```python
from build123d import *

# Parameters (mm, degrees)
SKETCH1_R             = 3.5
BOSS_EXTRUDE1_DEPTH   = 5
BOSS_EXTRUDE1_2_DEPTH = 5
BOSS_EXTRUDE1_3_DEPTH = 5
BOSS_EXTRUDE1_4_DEPTH = 5
SKETCH2_W             = 96.075
SKETCH2_H             = 46.545
BOSS_EXTRUDE3_DEPTH   = 1.5
SKETCH3_W             = 96.075
SKETCH3_H             = 46.545
SKETCH3_W_2           = 93.075
SKETCH3_H_2           = 43.545
BOSS_EXTRUDE4_DEPTH   = 10
FILLET1_R             = 3
FILLET2_R             = 1.5
FILLET3_R             = 2
FILLET4_R             = 0.5


with BuildPart() as part:
    # Sketch1 → Boss-Extrude1 (new body)
    with BuildSketch(Plane(origin=(0, 1.6, 0), x_dir=(1, 0, 0), z_dir=(0, 1, 0))):
        with Locations(Location((-41.5925, 16.8275, 0), (0, 0, 270))):
            Circle(SKETCH1_R)
    extrude(amount=BOSS_EXTRUDE1_DEPTH)



with BuildPart() as body_2:
    # Sketch1 → Boss-Extrude1 2 (new body)
    with BuildSketch(Plane(origin=(0, 1.6, 0), x_dir=(1, 0, 0), z_dir=(0, 1, 0))):
        with Locations(Location((-41.5925, -16.8275, 0), (0, 0, 270))):
            Circle(SKETCH1_R)
    extrude(amount=BOSS_EXTRUDE1_2_DEPTH)


with BuildPart() as body_3:
    # Sketch1 → Boss-Extrude1 3 (new body)
    with BuildSketch(Plane(origin=(0, 1.6, 0), x_dir=(1, 0, 0), z_dir=(0, 1, 0))):
        with Locations(Location((41.5925, -16.8275, 0), (0, 0, 270))):
            Circle(SKETCH1_R)
    extrude(amount=BOSS_EXTRUDE1_3_DEPTH)


with BuildPart() as body_4:
    # Sketch1 → Boss-Extrude1 4 (new body)
    with BuildSketch(Plane(origin=(0, 1.6, 0), x_dir=(1, 0, 0), z_dir=(0, 1, 0))):
        with Locations(Location((41.5925, 16.8275, 0), (0, 0, 270))):
            Circle(SKETCH1_R)
    extrude(amount=BOSS_EXTRUDE1_4_DEPTH)


with BuildPart() as part_1:
    add(part.part)

    add(body_2.part)  # Boss-Extrude3 merges body 2

    add(body_3.part)  # Boss-Extrude3 merges body 3

    add(body_4.part)  # Boss-Extrude3 merges body 4
    # Sketch2 → Boss-Extrude3 (add)
    with BuildSketch(Plane(origin=(0, 6.6, 0), x_dir=(1, 0, 0), z_dir=(0, 1, 0))):
        Rectangle(SKETCH2_W, SKETCH2_H)
    extrude(amount=-BOSS_EXTRUDE3_DEPTH)

    # Sketch3 → Boss-Extrude4 (add)
    with BuildSketch(Plane.XZ.offset(-5.1)):
        Rectangle(SKETCH3_W, SKETCH3_H)
        Rectangle(SKETCH3_W_2, SKETCH3_H_2, mode=Mode.SUBTRACT)
    extrude(amount=BOSS_EXTRUDE4_DEPTH)

    # Fillet1
    fillet1_edges = [part_1.edges().sort_by_distance(p)[0] for p in [
        (48.0375, 0.85, -23.2725),
        (48.0375, 0.85, 23.2725),
        (-48.0375, 0.85, 23.2725),
        (-48.0375, 0.85, -23.2725),
    ]]
    fillet(fillet1_edges, radius=FILLET1_R)

    # Fillet2
    fillet2_edges = [part_1.edges().sort_by_distance(p)[0] for p in [
        (46.5375, 0.1, -21.7725),
        (46.5375, 0.1, 21.7725),
        (-46.5375, 0.1, 21.7725),
        (-46.5375, 0.1, -21.7725),
    ]]
    fillet(fillet2_edges, radius=FILLET2_R)

    # Fillet3
    fillet3_edges = [part_1.edges().sort_by_distance(p)[0] for p in [
        (48.0375, 6.6, 0),
        (0, 6.6, -23.2725),
        (-48.0375, 6.6, 0),
        (0, 6.6, 23.2725),
        (47.158820344, 6.6, 22.393820344),
        (-47.158820344, 6.6, 22.393820344),
        (-47.158820344, 6.6, -22.393820344),
        (47.158820344, 6.6, -22.393820344),
    ]]
    fillet(fillet3_edges, radius=FILLET3_R)

    # Fillet4
    fillet4_edges = [part_1.edges().sort_by_distance(p)[0] for p in [
        (-46.5375, 5.1, 0),
        (0, 5.1, -21.7725),
        (46.5375, 5.1, 0),
        (0, 5.1, 21.7725),
        (46.098160172, 5.1, 21.333160172),
        (46.098160172, 5.1, -21.333160172),
        (-46.098160172, 5.1, 21.333160172),
        (-46.098160172, 5.1, -21.333160172),
    ]]
    fillet(fillet4_edges, radius=FILLET4_R)


solid = part_1.part
```
Source: CAD feature listing. Evaluate the final solid. Frame: model axes, mm. A direction names the side the tool comes from. Round coordinates to 2 decimals unless told otherwise and drop trailing zeros. Loops run counter-clockwise (first coordinate to the right, second up) from the corner with the lowest first, then second, coordinate; pieces in that order, holes last. Notation, with made-up numbers: M 23.5,46.5 L 73.5,46.5 A7 ccw 73.5,55.5 Z; hole C -2.75,49 d8. An arc over 180 degrees is marked long. Use a Markdown table: item, result. Add a question column.
1. Mould query, pull axis X, two halves, no side actions, for faces 3 (the cylindrical face through (47.467, 5.999, -0.284)), 4 (the cylindrical face through (-0.6, 6, -22.7)), 5 (the flat face through (46.538, 0, 0)), 6 (the flat face through (-48.038, 0, 0)). Classes: pulls with the +X half, pulls with the -X half, needs draft (parallel to the pull), parting line crosses it, or undercut.
2. Section query C-C on x = 12. Return the cut outline in (y, z).
3. Line query: line 1 (X direction, y = 0.25, z = 18); line 2 (Z direction, x = 32, y = 1.25); line 3 (X direction, y = 2.25, z = 14.5). Output: solid intervals per line, ascending.
4. Section query A-A on z = -2.5. Return the cut outline in (x, y).
5. Reachability of faces 1 (the cylindrical face through (-47.467, 5.999, 0.284)), 2 (the cylindrical face through (38.176, 3.326, 16.069)) from +Z, -Z, +X, -X, +Y, -Y: full face, straight path, thin tool, end or side. Return the list, or none.
6. Section query B-B on y = 2.5. Return the cut outline in (x, z).
7. Contact query for flat-ended pins moving along their axis: P1, Ø3.5, axis at x = -42, z = 16.5, coming from the -Y side; P2, Ø2, axis at x = -31, z = -2.5, coming from the -Y side; P3, Ø1.5, axis at y = 5.5, z = -15, coming from the +X side. Output: stop coordinate, or through.
8. Section query D-D on y = -3.25. Return the cut outline in (x, z).
Reported:
| question | item | result |
|---|---|---|
| 1 | face 3 | pulls with the +X half |
| 1 | face 4 | needs draft |
| 1 | face 5 | undercut |
| 1 | face 6 | pulls with the -X half |
| 2 | outline | M -4.9,-23.27 L 4.6,-23.27 A2 ccw 6.6,-21.27 L 6.6,21.27 A2 ccw 4.6,23.27 L -4.9,23.27 L -4.9,21.77 L 4.6,21.77 A0.5 cw 5.1,21.27 L 5.1,-21.27 A0.5 cw 4.6,-21.77 L -4.9,-21.77 Z |
| 3 | line 1 | x = -48.04 to -46.54, 46.54 to 48.04 |
| 3 | line 2 | z = -23.27 to -21.77, 21.77 to 23.27 |
| 3 | line 3 | x = -48.04 to -46.54, -44.21 to -38.98, 38.98 to 44.21, 46.54 to 48.04 |
| 4 | outline | M -48.04,-4.9 L -46.54,-4.9 L -46.54,4.6 A0.5 cw -46.04,5.1 L 46.04,5.1 A0.5 cw 46.54,4.6 L 46.54,-4.9 L 48.04,-4.9 L 48.04,4.6 A2 ccw 46.04,6.6 L -46.04,6.6 A2 ccw -48.04,4.6 Z |
| 5 | face 1 | +Z, -Z, -X, +Y |
| 5 | face 2 | -Y |
| 6 | outline | M -48.04,-20.27 A3 ccw -45.04,-23.27 L 45.04,-23.27 A3 ccw 48.04,-20.27 L 48.04,20.27 A3 ccw 45.04,23.27 L -45.04,23.27 A3 ccw -48.04,20.27 Z; C -41.59,-16.83 d7; C -41.59,16.83 d7; C 41.59,-16.83 d7; C 41.59,16.83 d7; hole M -46.54,-20.27 A1.5 ccw -45.04,-21.77 L 45.04,-21.77 A1.5 ccw 46.54,-20.27 L 46.54,20.27 A1.5 ccw 45.04,21.77 L -45.04,21.77 A1.5 ccw -46.54,20.27 Z |
| 7 | P1 | stops at y = 1.6 |
| 7 | P2 | stops at y = 5.1 |
| 7 | P3 | stops at x = 48.03 |
| 8 | outline | M -48.04,-20.27 A3 ccw -45.04,-23.27 L 45.04,-23.27 A3 ccw 48.04,-20.27 L 48.04,20.27 A3 ccw 45.04,23.27 L -45.04,23.27 A3 ccw -48.04,20.27 Z; hole M -46.54,-20.27 A1.5 ccw -45.04,-21.77 L 45.04,-21.77 A1.5 ccw 46.54,-20.27 L 46.54,20.27 A1.5 ccw 45.04,21.77 L -45.04,21.77 A1.5 ccw -46.54,20.27 Z |
